CAD build for the part. Positions are in the model's coordinates, mm. Round coordinates to 2 decimals unless told otherwise and drop trailing zeros. Write each loop counter-clockwise with the first axis right and the second up, starting at its lowest first coordinate (ties: lowest second). Pieces come first, ordered by that corner, then holes. Notation, with made-up numbers: (23.25, -22.5) - (53.25, -22.5) arc R18 ccw to (53.25, -6.5) - close; hole circle Ø11 at (22, 12). An arc over 180 degrees is marked (long way). Answer in a Markdown table with one row per item.
```python
from build123d import *

# Parameters (mm, degrees)
SKETCH1_R             = 100
SKETCH1_R_2           = 40
SKETCH1_R_3           = 3.05
BOSS_EXTRUDE1_DEPTH   = 15
SKETCH2_R             = 3
CUT_EXTRUDE1_DEPTH    = 143.214626533
CIRPATTERN1_COUNT     = 6
CIRPATTERN2_OUTLINE_R = 3.05
CIRPATTERN2_DEPTH     = 15


# Read off the part's stored shape, not the designer's step: CirPattern2
with BuildPart() as part:
    # Sketch1 → Boss-Extrude1 (new body)
    with BuildSketch(Plane(origin=(0, 0, 0), x_dir=(1, 0, 0), z_dir=(0, 1, 0))):
        with Locations(Location((0, 0, 0), (0, 0, 270))):
            Circle(SKETCH1_R)
        with Locations(Location((0, 0, 0), (0, 0, 270))):
            Circle(SKETCH1_R_2, mode=Mode.SUBTRACT)
        with Locations(Location((12.723046489, -48.354152749, 0), (0, 0, 270))):
            Circle(SKETCH1_R_3, mode=Mode.SUBTRACT)
    extrude(amount=BOSS_EXTRUDE1_DEPTH)

    # Sketch2 → Cut-Extrude1 (cut, through all)
    with BuildSketch(Plane(origin=(0, 0, 0), x_dir=(0, 0, -1), z_dir=(1, 0, 0))):
        with Locations((0, 7.5)):
            Circle(SKETCH2_R)
    cut_extrude1 = extrude(amount=-CUT_EXTRUDE1_DEPTH, mode=Mode.SUBTRACT)

    # CirPattern1: Cut-Extrude1 ×6 about axis
    cirpattern1_axis = Axis((0, 15, 0), (0, 1, 0))
    for i in range(1, CIRPATTERN1_COUNT):
        add(cut_extrude1.rotate(cirpattern1_axis, i * 360 / CIRPATTERN1_COUNT), mode=Mode.SUBTRACT)

    # CirPattern2 outline → CirPattern2 (cut)
    with BuildSketch(Plane(origin=(0, 0, 0), x_dir=(1, 0, 0), z_dir=(0, 1, 0))):
        with Locations((-35.514401414, -35.195557847)):
            Circle(CIRPATTERN2_OUTLINE_R)
        with Locations((-48.237447903, 13.158594901)):
            Circle(CIRPATTERN2_OUTLINE_R)
        with Locations((-12.723046489, 48.354152749)):
            Circle(CIRPATTERN2_OUTLINE_R)
        with Locations((35.514401414, 35.195557847)):
            Circle(CIRPATTERN2_OUTLINE_R)
        with Locations((48.237447903, -13.158594901)):
            Circle(CIRPATTERN2_OUTLINE_R)
    extrude(amount=CIRPATTERN2_DEPTH, mode=Mode.SUBTRACT)


solid = part.part
```
Q1. Saw through at B-B on z = 0. List the corners of the cut face in (x, y), then the cut area to 3 significant figures.
Computed:
| item | result |
|---|---|
| outline | (-100, 0) - (-40, 0) - (-40, 4.5) - (-100, 4.5) - close; (-100, 10.5) - (-40, 10.5) - (-40, 15) - (-100, 15) - close; (40, 0) - (100, 0) - (100, 4.5) - (40, 4.5) - close; (40, 10.5) - (100, 10.5) - (100, 15) - (40, 15) - close |
| area | 1,080 mm2 |
Q2. Drill centre lines: line 1 (X direction, y = 10, z = -75); line 2 (X direction, y = 6.5, z = -73); line 3 (Z direction, x = -33, y = 2). Where is each one in solid material? Low to high.
Computed:
| item | result |
|---|---|
| line 1 | x = -66.14 to -45.22, -41.39 to 41.39, 45.22 to 66.14 |
| line 2 | x = -68.34 to -45.41, -38.88 to 38.88, 45.41 to 68.34 |
| line 3 | z = -94.4 to -22.61, 22.61 to 33.47, 36.92 to 94.4 |
Q3. Pull direction Y, two halves, no side cores. Call faces 1 (the cylindrical face through (-69.5, 7.6, 3)), 2 (the flat face through (-43, 0, -1)), 3 (the cylindrical face through (-46.6, 7.4, -15.73)): released by +Y, released by -Y, zero draft, split by the parting line, or undercut.
Computed:
| item | result |
|---|---|
| face 1 | undercut |
| face 2 | released by -Y |
| face 3 | zero draft |
Q4. Saw through at A-A on x = 0. List the corners of the cut face in (y, z), then the cut area to 3 significant figures.
Computed:
| item | result |
|---|---|
| outline | (0, -100) - (15, -100) - (15, -40) - (0, -40) - close; (0, 40) - (15, 40) - (15, 100) - (0, 100) - close |
| area | 1,800 mm2 |
Q5. Saw through at C-C on y = 7.5. Count the separate pieces of the cut face and the enclosed holes in it, then the cut area to 3 significant figures.
Computed:
| item | result |
|---|---|
| separate pieces | 6 |
| enclosed holes | 6 |
| area | 24,100 mm2 |
Q6. Flat gauge pins, fed straight in: pin 1 (5 mm diameter, centred on x = -12.72, z = -48.35, fed in from +Y); pin 2 (6 mm diameter, centred on x = -28, y = 2, fed in from +Z); pin 3 (6 mm diameter, centred on x = 46.5, y = 5, fed in from +Z); pin 4 (2 mm diameter, centred on y = 5, z = 63.5, fed in from +X). Where does each tip first touch, or does it go through?
Computed:
| item | result |
|---|---|
| pin 1 | passes through |
| pin 2 | stops at z = 96.82 |
| pin 3 | stops at z = 90.04 |
| pin 4 | stops at x = 78.06 |
